Geometry check sheet. Reference: the model listing, model coordinates, mm. A direction names the side the tool comes from. Give positions to 0.01 mm unless a question says otherwise; leave off trailing zeros. Write each loop counter-clockwise with the first axis right and the second up, starting at its lowest first coordinate (ties: lowest second). Pieces come first, ordered by that corner, then holes. Notation, with made-up numbers: (50, 41.5) - (101, 41.5) arc R36 ccw to (101, 77.5) - close; hole circle Ø2 at (79, -25). An arc over 180 degrees is marked (long way). Write item = value, one per line. Start each with the question number.
(1) Section check B-B, the plane z = 3. Give the number of separate pieces and of enclosed holes in the cut face, plus the area to 3 significant figures.
(2) Depth check by flat-ended pin: pin 1 Ø9 at (x, y) = (25.5, 68.5) entering from +Z; pin 2 Ø4 at (x, y) = (72, 78.5) entering from -Z; pin 3 Ø5 at (y, z) = (69, 16) entering from +X. Enter the tip coordinate at first touch or a pass-through.
(3) Section check A-A, the plane z = 56.5. Enter the section's corners in (x, y).
(4) Access from +Z, -Z, +X, -X, +Y, -Y to the whole of each face (thin tool, end or side, straight path). Record for faces 1 (the cylindrical face through (119.575, 52.974, 77.535)), 2 (the flat face through (0, 47.7, 70.2)), 3 (the flat face through (0, 48, -7)).
(5) Draft check along Z on faces 4 (the flat face through (33, 65, 5)), 5 (the flat face through (-2, 87, 24)), 6 (the cylindrical face through (128.19, 30.76, 42.54)). Enter one of: pulls with the +Z half, pulls with the -Z half, needs draft (parallel to the pull), parting line crosses it, or undercut.
(6) Thickness scan on L1, parallel to Z at x = 6.5, y = 30.5; L2, parallel to Y at x = 111, z = 43; L3, parallel to Y at x = 154.5, z = 3.7. Record the ranges inside material, lowest first.
```python
from build123d import *

# Parameters (mm, degrees)
F0_W           = 180
F0_H           = 94
F1_DEPTH       = 80
F2_R           = 17.5
F3_DEPTH       = 75
F4_W           = 94
F4_H           = 30
F5_DEPTH       = 180.001
F6_W           = 94
F6_H           = 100
F7_DEPTH       = 5
F8_W           = 94
F8_H           = 100
F9_DEPTH       = 5
F10_R          = 7.5
F11_DEPTH      = 25
F12_W          = 80
F12_H          = 18
F13_DEPTH      = 5.001
F13_DEPTH_BACK = 185.001


with BuildPart() as f1:
    # F0 (on Top) → F1 (new body)
    with BuildSketch(Plane.XY):
        with Locations((90, 47)):
            Rectangle(F0_W, F0_H)
    extrude(amount=F1_DEPTH)

    # F2 (on face) → F3 (cut)
    with BuildSketch(Plane.XY.offset(80)):
        with Locations((25.5, 25.5)):
            Circle(F2_R)
        with Locations((25.5, 68.5)):
            Circle(F2_R)
        with Locations((68.5, 25.5)):
            Circle(F2_R)
        with Locations((68.5, 68.5)):
            Circle(F2_R)
        with Locations((111.5, 25.5)):
            Circle(F2_R)
        with Locations((111.5, 68.5)):
            Circle(F2_R)
        with Locations((154.5, 25.5)):
            Circle(F2_R)
        with Locations((154.5, 68.5)):
            Circle(F2_R)
    extrude(amount=-F3_DEPTH, mode=Mode.SUBTRACT)

    # F4 (on face) → F5 (cut, through all)
    with BuildSketch(Plane.YZ.offset(180)):
        with Locations((47, 60)):
            Rectangle(F4_W, F4_H)
        with Locations((47, 25)):
            Rectangle(F4_W, F4_H)
    extrude(amount=-F5_DEPTH, mode=Mode.SUBTRACT)

    # F6 (on face) → F7 (join)
    with BuildSketch(Plane(origin=(0, 0, 0), x_dir=(0, -1, 0), z_dir=(-1, 0, 0))):
        with Locations((-47, 35)):
            Rectangle(F6_W, F6_H)
    extrude(amount=F7_DEPTH)

    # F8 (on face) → F9 (join)
    with BuildSketch(Plane.YZ.offset(180)):
        with Locations((47, 35)):
            Rectangle(F8_W, F8_H)
    extrude(amount=F9_DEPTH)

    # F10 (on face) → F11 (cut)
    with BuildSketch(Plane.XY.offset(5)):
        with Locations((25.5, 25.5)):
            Circle(F10_R)
        with Locations((25.5, 68.5)):
            Circle(F10_R)
        with Locations((68.5, 25.5)):
            Circle(F10_R)
        with Locations((68.5, 68.5)):
            Circle(F10_R)
        with Locations((111.5, 25.5)):
            Circle(F10_R)
        with Locations((111.5, 68.5)):
            Circle(F10_R)
        with Locations((154.5, 25.5)):
            Circle(F10_R)
        with Locations((154.5, 68.5)):
            Circle(F10_R)
    extrude(amount=-F11_DEPTH, mode=Mode.SUBTRACT)

    # F12 (on face) → F13 (cut, two sides)
    with BuildSketch(Plane(origin=(180, 0, 0), x_dir=(0, -1, 0), z_dir=(-1, 0, 0))) as f13_sk:
        with Locations((-47, 61)):
            Rectangle(F12_W, F12_H)
        with Locations((-47, 24)):
            Rectangle(F12_W, F12_H)
    extrude(amount=-F13_DEPTH, mode=Mode.SUBTRACT)
    extrude(f13_sk.sketch, amount=F13_DEPTH_BACK, mode=Mode.SUBTRACT)


solid = f1.part
```
Model answer:
q1.separate_pieces = 1
q1.enclosed_holes = 8
q1.area = 16,400 mm²
q2.pin_1 = through
q2.pin_2 = 0
q2.pin_3 = 185
q3.outline = (-5, 0) - (0, 0) - (0, 7) - (-5, 7) - close; (-5, 87) - (0, 87) - (0, 94) - (-5, 94) - close; (180, 0) - (185, 0) - (185, 7) - (180, 7) - close; (180, 87) - (185, 87) - (185, 94) - (180, 94) - close
q4.face_1 = +Z
q4.face_2 = +Y, -Y
q4.face_3 = -Z, +Y, -Y
q5.face_4 = pulls with the +Z half
q5.face_5 = undercut
q5.face_6 = needs draft
q6.L1 = 0 to 10, 40 to 45, 75 to 80
q6.L2 = 0 to 8.01, 42.99 to 51.01, 85.99 to 94
q6.L3 = 0 to 18, 33 to 61, 76 to 94
